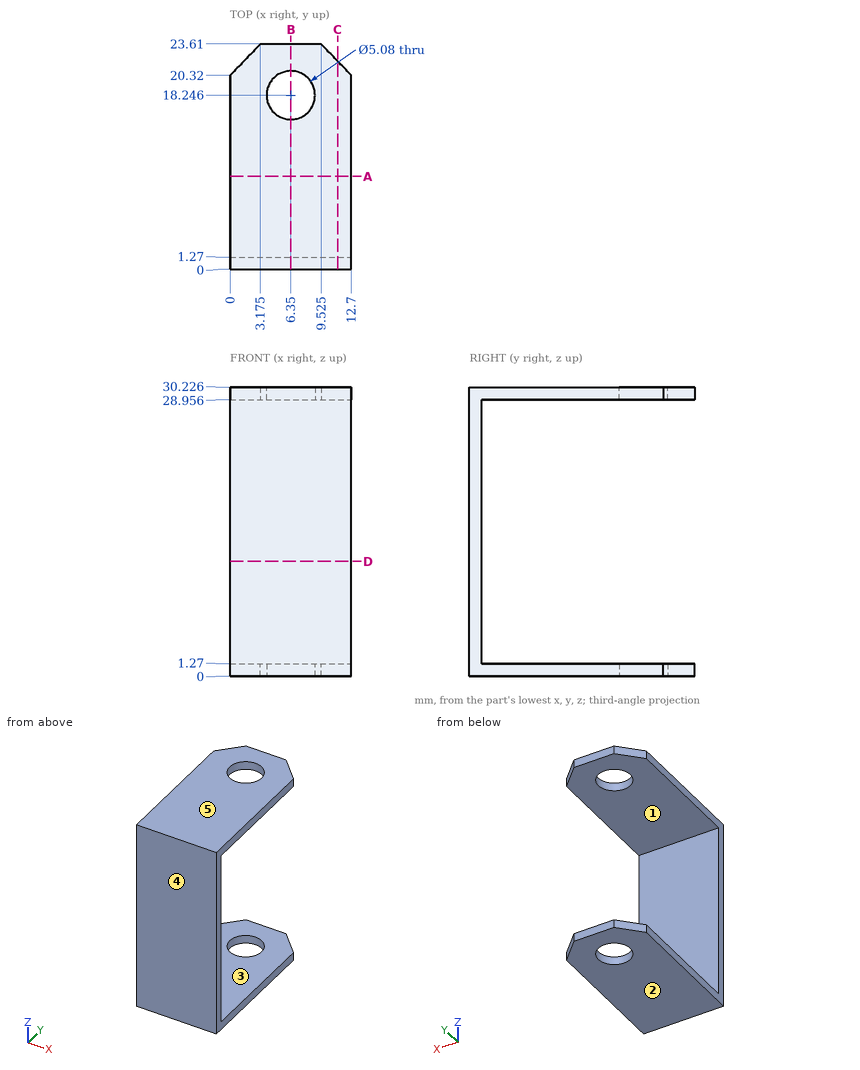
Geometry check sheet. Reference: drawing and pictorial views, mm from the part's lowest x, y, z. A direction names the side the tool comes from. Round coordinates to 2 decimals unless told otherwise and drop trailing zeros. Order: outer loops, then holes, each group sorted by start corner. A loop starts at its lowest first (then second) coordinate and runs counter-clockwise, first axis right, second up. Notation, with made-up numbers: (48, -22) -> (65, -22) arc R17 cw to (65, -18) -> close; hole circle Ø4 at (40.5, 40.25). An arc over 180 degrees is marked (long way). One line per item, written item: value. Start each with the question number.
Q1. Gauge pin test, flat ends, axial feed: pin 1 Ø4 at (x, y) = (6.35, 18.25) entering from -Z; pin 2 Ø3 at (x, z) = (8, 24.5) entering from +Y. Record the tip position at first contact, or that the pin passes through.
Q2. Cross-section at C-C (x = 11.25). Record the boundary of the cut face in (y, z).
Q3. Cross-section at D-D (z = 12). Record the boundary of the cut face in (x, y), and give its area (3 significant figures).
Q4. Mould release check, pull along Z, two halves, no side actions. Record for the marked faces 3, 4 and 5: pulls with the +Z half, pulls with the -Z half, needs draft (parallel to the pull), parting line crosses it, or undercut.
Q5. Thickness scan on line 1 (Y direction, x = 6.35, z = 0.65); line 2 (Z direction, x = 7.5, y = 21.5); line 3 (Y direction, x = 7.75, z = 7). Record the ranges inside material, lowest first.
Q6. Cross-section at A-A (y = 9.75). Record the boundary of the cut face in (x, z).
Q7. Set-up check for the marked faces 1 and 2: record each of +Z, -Z, +X, -X, +Y, -Y from which the full face is reachable in a straight line by a thin tool's end or side.
Q8. Cross-section at B-B (x = 6.35). Record the boundary of the cut face in (y, z).
Completed:
1. pin 1: passes through
1. pin 2: stops at y = 1.27
2. outline: (0, 0) -> (21.82, 0) -> (21.82, 1.27) -> (1.27, 1.27) -> (1.27, 28.96) -> (21.82, 28.96) -> (21.82, 30.23) -> (0, 30.23) -> close
3. outline: (0, 0) -> (12.7, 0) -> (12.7, 1.27) -> (0, 1.27) -> close
3. area: 16.1 mm²
4. face 3: undercut
4. face 4: needs draft
4. face 5: pulls with the +Z half
5. line 1: y = 0 to 15.71, 20.79 to 23.61
5. line 2: z = 0 to 1.27, 28.96 to 30.23
5. line 3: y = 0 to 1.27
6. outline: (0, 0) -> (12.7, 0) -> (12.7, 1.27) -> (0, 1.27) -> close; (0, 28.96) -> (12.7, 28.96) -> (12.7, 30.23) -> (0, 30.23) -> close
7. face 1: +X, -X, +Y
7. face 2: -Z, +X, -X, +Y, -Y
8. outline: (0, 0) -> (15.71, 0) -> (15.71, 1.27) -> (1.27, 1.27) -> (1.27, 28.96) -> (15.71, 28.96) -> (15.71, 30.23) -> (0, 30.23) -> close; (20.79, 0) -> (23.61, 0) -> (23.61, 1.27) -> (20.79, 1.27) -> close; (20.79, 28.96) -> (23.61, 28.96) -> (23.61, 30.23) -> (20.79, 30.23) -> close
